The model under review builds one solid part; all positions refer to its coordinate system, in mm. A direction names the side the tool comes from. Give positions to 0.01 mm unless a question says otherwise; leave off trailing zeros. Order: outer loops, then holes, each group sorted by start corner. A loop starts at its lowest first (then second) coordinate and runs counter-clockwise, first axis right, second up. Notation, with made-up numbers: (71.5, 83.25) - (110.5, 83.25) arc R18 ccw to (110.5, 114.25) - close; hole circle Ø3 at (28.5, 9). An arc over 180 degrees is marked (long way). Answer as CSV lines item,"result". Start each with the question number.
from build123d import *

# Parameters (mm, degrees)
SKETCH1_W               = 494
SKETCH1_H               = 33
BOSS_EXTRUDE2_DEPTH     = 166
SKETCH6_W               = 494
SKETCH6_H               = 32.558092213
CUT_EXTRUDE2_DEPTH      = 156
SKETCH8_W               = 494
SKETCH8_H               = 30
BOSS_EXTRUDE3_DEPTH     = 2.5
SKETCH9_W               = 494
SKETCH9_H               = 30
BOSS_EXTRUDE4_DEPTH     = 2.5
SKETCH10_W              = 494
SKETCH10_H              = 30
BOSS_EXTRUDE5_DEPTH     = 2.5
SKETCH11_W              = 494
SKETCH11_H              = 30
BOSS_EXTRUDE6_DEPTH     = 2.5
SKETCH7_R               = 3
SKETCH7_R_2             = 2
SKETCH7_R_3             = 2.270552225
CUT_EXTRUDE3_DEPTH      = 1
CUT_EXTRUDE3_DEPTH_BACK = 81.774674129


with BuildPart() as part:
    # Sketch1 → Boss-Extrude2 (new body, symmetric)
    with BuildSketch(Plane.XY):
        with BuildLine():
            Line((0, 0), (0, 49))
            Line((0, 49), (500, 49))
            Line((500, 49), (500, 0))
            ThreePointArc((500, 0), (250, -31.774674129), (0, 0))
        make_face()
        with Locations((250, 29)):
            Rectangle(SKETCH1_W, SKETCH1_H, mode=Mode.SUBTRACT)
    extrude(amount=BOSS_EXTRUDE2_DEPTH, both=True)

    # Sketch6 → Cut-Extrude2 (cut, symmetric)
    with BuildSketch(Plane.XY):
        with Locations((250, -16.279046107)):
            Rectangle(SKETCH6_W, SKETCH6_H)
    extrude(amount=CUT_EXTRUDE2_DEPTH, both=True, mode=Mode.SUBTRACT)

    # Sketch8 → Boss-Extrude3 (add)
    with BuildSketch(Plane(origin=(0, 12.5, 0), x_dir=(1, 0, 0), z_dir=(0, 1, 0))):
        with Locations((250, -151)):
            Rectangle(SKETCH8_W, SKETCH8_H)
    extrude(amount=BOSS_EXTRUDE3_DEPTH)

    # Sketch9 → Boss-Extrude4 (add)
    with BuildSketch(Plane.XZ.offset(-45.5)):
        with Locations((250, 151)):
            Rectangle(SKETCH9_W, SKETCH9_H)
    extrude(amount=BOSS_EXTRUDE4_DEPTH)

    # Sketch10 → Boss-Extrude5 (add)
    with BuildSketch(Plane.XZ.offset(-45.5)):
        with Locations((250, -151)):
            Rectangle(SKETCH10_W, SKETCH10_H)
    extrude(amount=BOSS_EXTRUDE5_DEPTH)

    # Sketch11 → Boss-Extrude6 (add)
    with BuildSketch(Plane(origin=(0, 12.5, 0), x_dir=(1, 0, 0), z_dir=(0, 1, 0))):
        with Locations((250, 151)):
            Rectangle(SKETCH11_W, SKETCH11_H)
    extrude(amount=BOSS_EXTRUDE6_DEPTH)

    # Sketch7 → Cut-Extrude3 (cut, two sides)
    with BuildSketch(Plane(origin=(0, 49, 0), x_dir=(1, 0, 0), z_dir=(0, 1, 0))) as cut_extrude3_sk:
        with Locations((230, -146)):
            Circle(SKETCH7_R)
        with Locations((300, -146)):
            Circle(SKETCH7_R)
        with Locations((370, -146)):
            Circle(SKETCH7_R)
        with Locations((440, -146)):
            Circle(SKETCH7_R)
        with Locations((231.366830489, -152.86525851)):
            Circle(SKETCH7_R_2)
        with Locations((301.366830489, -152.86525851)):
            Circle(SKETCH7_R_3)
        with Locations((371.366830489, -152.86525851)):
            Circle(SKETCH7_R_2)
        with Locations((441.366830489, -152.86525851)):
            Circle(SKETCH7_R_2)
        with Locations((237, -146)):
            Circle(SKETCH7_R_2)
        with Locations((307, -146)):
            Circle(SKETCH7_R_2)
        with Locations((377, -146)):
            Circle(SKETCH7_R_2)
        with Locations((447, -146)):
            Circle(SKETCH7_R_2)
        with Locations((440, 146)):
            Circle(SKETCH7_R)
        with Locations((370, 146)):
            Circle(SKETCH7_R)
        with Locations((300, 146)):
            Circle(SKETCH7_R)
        with Locations((230, 146)):
            Circle(SKETCH7_R)
        with Locations((441.366830489, 152.86525851)):
            Circle(SKETCH7_R_2)
        with Locations((447, 146)):
            Circle(SKETCH7_R_2)
        with Locations((371.366830489, 152.86525851)):
            Circle(SKETCH7_R_2)
        with Locations((377, 146)):
            Circle(SKETCH7_R_2)
        with Locations((307, 146)):
            Circle(SKETCH7_R_2)
        with Locations((301.366830489, 152.86525851)):
            Circle(SKETCH7_R_3)
        with Locations((237, 146)):
            Circle(SKETCH7_R_2)
        with Locations((231.366830489, 152.86525851)):
            Circle(SKETCH7_R_2)
    extrude(amount=CUT_EXTRUDE3_DEPTH, mode=Mode.SUBTRACT)
    extrude(cut_extrude3_sk.sketch, amount=-CUT_EXTRUDE3_DEPTH_BACK, mode=Mode.SUBTRACT)


solid = part.part
Item 1: Take a section at A-A on z = 46.5. Write out the cut boundary in (x, y) (3 decimals), and give its area (3 significant figures).
Item 2: Mouldability with a two-part tool opening along X and no side actions: class faces 4 (the face through (247, 15, -151)), 5 (the face through (251.179, -31.774, 160.627)), 6 (the face through (500, 25, 2)), 7 (the face through (3, 29, 2)) as released by +X, released by -X, zero draft, split by the parting line, or undercut.
Item 3: Clearance check with flat-ended pins moving along their axes: pin 1 (3 mm diameter, centred on y = 37.5, z = 103, fed in from -X); pin 2 (5 mm diameter, centred on x = 216, z = -40.5, fed in from -Y). State where each tip first meets the part, or that it passes through.
Item 4: Take a section at D-D on x = 147.5. Write out the cut boundary in (y, z).
Item 5: For line 1 along Y through (x, z) = (381, 128); line 2 along X through (y, z) = (29, -53); line 3 along Z through (x, y) = (447, 8), list the stretches that pass through material, from the lowest coordinate up.
Item 6: Take a section at B-B on x = 400. Write out the cut boundary in (y, z), and give its area (3 significant figures).
Item 7: Machinability: for faces 1 (the face through (247, 0, 2)), 2 (the face through (247, 43, 151)), 3 (the face through (247, 45.5, 2)), which of the approach directions +Z, -Z, +X, -X, +Y, -Y give a long, thin tool a straight path to every point of the face, cutting with its end or side? Answer none if there is none.
Data:
1,outline,"(0, 0) arc R999.375 ccw to (3, -0.77) - (3, 0) - (497, 0) - (497, -0.77) arc R999.375 ccw to (500, 0) - (500, 49) - (0, 49) - close; hole (3, 12.5) - (497, 12.5) - (497, 45.5) - (3, 45.5) - close"
1,area,"8,200 mm^2"
2,face 4,"undercut"
2,face 5,"split by the parting line"
2,face 6,"released by +X"
2,face 7,"undercut"
3,pin 1,"stops at x = 0"
3,pin 2,"stops at y = 0"
4,outline,"(-26.5, -166) - (15, -166) - (15, -136) - (12.5, -136) - (12.5, 136) - (15, 136) - (15, 166) - (-26.5, 166) - (-26.5, 156) - (0, 156) - (0, -156) - (-26.5, -156) - close; (43, -166) - (49, -166) - (49, 166) - (43, 166) - (43, 136) - (45.5, 136) - (45.5, -136) - (43, -136) - close"
5,line 1,"y = 0 to 12.5, 45.5 to 49"
5,line 2,"x = 0 to 3, 497 to 500"
5,line 3,"z = -166 to -148, -144 to 144, 148 to 166"
6,outline,"(-20.45, -166) - (15, -166) - (15, -136) - (12.5, -136) - (12.5, 136) - (15, 136) - (15, 166) - (-20.45, 166) - (-20.45, 156) - (0, 156) - (0, -156) - (-20.45, -156) - close; (43, -166) - (49, -166) - (49, 166) - (43, 166) - (43, 136) - (45.5, 136) - (45.5, -136) - (43, -136) - close"
6,area,"6,020 mm^2"
7,face 1,"-Y"
7,face 2,"+Z, -Z"
7,face 3,"none"
